```python
from build123d import *

# Parameters (mm, degrees)
BOSS_EXTRUDE1_DEPTH = 5
SKETCH2_R           = 2
CUT_EXTRUDE1_DEPTH  = 5
SKETCH3_W           = 90
SKETCH3_H           = 10
SKETCH3_H_2         = 50
CUT_EXTRUDE2_DEPTH  = 5


with BuildPart() as part:
    # Sketch1 → Boss-Extrude1 (new body)
    with BuildSketch(Plane.XY):
        Polygon((-70, -15), (-70, -63.64), (70, -63.64), (70, -15), (75, -15), (75, 15), (70, 15), (70, 63.64), (-70, 63.64), (-70, 15), (-75, 15), (-75, -15), align=None)
    extrude(amount=BOSS_EXTRUDE1_DEPTH)

    # Sketch2 → Cut-Extrude1 (cut)
    with BuildSketch(Plane.XY.offset(5)):
        with Locations((-72.5, 0)):
            Circle(SKETCH2_R)
        with Locations((72.5, 0)):
            Circle(SKETCH2_R)
    extrude(amount=-CUT_EXTRUDE1_DEPTH, mode=Mode.SUBTRACT)

    # Sketch3 → Cut-Extrude2 (cut)
    with BuildSketch(Plane.XY.offset(5)):
        with Locations((-15, 58.64)):
            Rectangle(SKETCH3_W, SKETCH3_H)
        with Locations((-15, -38.64)):
            Rectangle(SKETCH3_W, SKETCH3_H_2)
    extrude(amount=-CUT_EXTRUDE2_DEPTH, mode=Mode.SUBTRACT)


solid = part.part
```
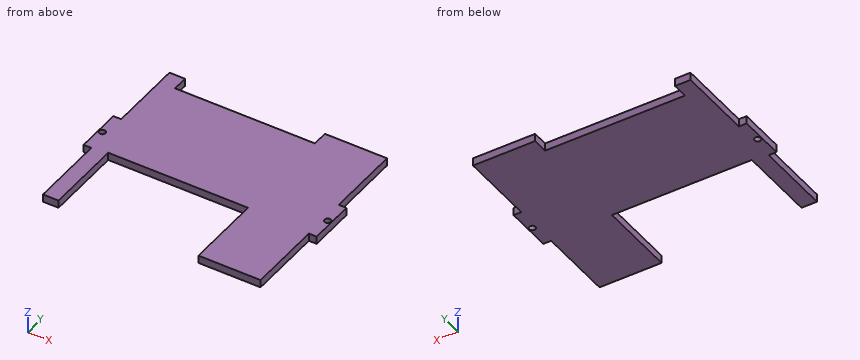
Geometry: final body of the model. Coordinates: model frame, mm. Coordinates: 2 decimals unless noted, no trailing zeros. Order: outer loops, then holes, each group sorted by start corner. A loop starts at its lowest first (then second) coordinate and runs counter-clockwise, first axis right, second up. Notation, with made-up numbers: (-32.75, -9.75) - (-6.75, -9.75) arc R24 cw to (-6.75, 10.25) - close; hole circle Ø4 at (88, 82.25). An arc over 180 degrees is marked (long way). Write each question's results on one line, items separated by ' | '.
(1) Section query C-C, the plane y = -52. Return the cut outline in (x, z).
Values found:
outline: (-70, 0) - (-60, 0) - (-60, 5) - (-70, 5) - close; (30, 0) - (70, 0) - (70, 5) - (30, 5) - close
(2) Section query D-D, the plane z = 2.5. Return the cut outline in (x, y).
Values found:
outline: (-75, -15) - (-70, -15) - (-70, -63.64) - (-60, -63.64) - (-60, -13.64) - (30, -13.64) - (30, -63.64) - (70, -63.64) - (70, -15) - (75, -15) - (75, 15) - (70, 15) - (70, 63.64) - (30, 63.64) - (30, 53.64) - (-60, 53.64) - (-60, 63.64) - (-70, 63.64) - (-70, 15) - (-75, 15) - close; hole circle Ø4 at (-72.5, 0); hole circle Ø4 at (72.5, 0)
(3) Section query A-A, the plane x = 72.5. Return the cut outline in (y, z), plus the area to 3 significant figures.
Values found:
outline: (-15, 0) - (-2, 0) - (-2, 5) - (-15, 5) - close; (2, 0) - (15, 0) - (15, 5) - (2, 5) - close | area: 130 mm²
(4) Line query: line 1 (Y direction, x = -72.5, z = 2.9); line 2 (X direction, y = 34.5, z = 2.45); line 3 (Y direction, x = -58, z = 1.2). Output: solid intervals per line, ascending. Write a range as [from, to].
Values found:
line 1: y = [-15, -2], [2, 15] | line 2: x = [-70, 70] | line 3: y = [-13.64, 53.64]
(5) First-contact query: pin 1 Ø2.5 at (y, z) = (-28, 3.5) entering from -X; pin 2 Ø2.5 at (y, z) = (-51.5, 3) entering from +X; pin 3 Ø2 at (x, z) = (-7.5, 2) entering from +Y. Flat tips, straight axial feed; report the tip coordinate or a pass-through.
Values found:
pin 1: stops at x = -70 | pin 2: stops at x = 70 | pin 3: stops at y = 53.64
(6) Section query B-B, the plane y = 0. Return the cut outline in (x, z).
Values found:
outline: (-75, 0) - (-74.5, 0) - (-74.5, 5) - (-75, 5) - close; (-70.5, 0) - (70.5, 0) - (70.5, 5) - (-70.5, 5) - close; (74.5, 0) - (75, 0) - (75, 5) - (74.5, 5) - close
